Part model, mm, in its own coordinate system. Coordinates: 2 decimals unless noted, no trailing zeros. Order: outer loops, then holes, each group sorted by start corner. A loop starts at its lowest first (then second) coordinate and runs counter-clockwise, first axis right, second up.
1) Cut at A-A (x = 0). List the corners of the cut face in (y, z).
2) Cut at D-D (z = -25). List the corners of the cut face in (x, y).
3) Cut at C-C (z = 8.5). List the corners of the cut face in (x, y), and give its area (3 significant figures).
4) Cut at B-B (z = 0). List the corners of the cut face in (x, y), and give its area (3 significant figures).
5) Pin check, flat tips, straight feed: pin 1 Ø4 at (x, z) = (21.65, 12.5) entering from +Y; pin 2 Ø1 at (x, y) = (23.5, 0.5) entering from -Z; pin 3 Ø6 at (x, z) = (0, -15.25) entering from -Y. Stop position of each tip, or through.
6) Wall check: L1, parallel to X at y = 2.6, z = -14; L2, parallel to X at y = 0.8, z = 10.5; L3, parallel to Z at x = -11.5, y = 2.5. Give the ranges that are in metal, low to high.
```python
from build123d import *

# Parameters (mm, degrees)
SKETCH1_R           = 30
SKETCH1_R_2         = 17
BOSS_EXTRUDE1_DEPTH = 3
SKETCH2_R           = 4.75
SKETCH2_R_2         = 2.55
BOSS_EXTRUDE2_DEPTH = 3
SKETCH3_R           = 2.55
CUT_EXTRUDE1_DEPTH  = 43.532340636
CIRPATTERN1_COUNT   = 3
FILLET1_R           = 0.5
SKETCH4_R           = 2.55
CUT_EXTRUDE2_DEPTH  = 43.532340784
CIRPATTERN2_COUNT   = 3


with BuildPart() as part:
    # Sketch1 → Boss-Extrude1 (new body)
    with BuildSketch(Plane(origin=(0, 0, 0), x_dir=(1, 0, 0), z_dir=(0, 1, 0))):
        with Locations(Location((0, 0, 0), (0, 0, 270))):
            Circle(SKETCH1_R)
        with Locations(Location((0, 0, 0), (0, 0, 270))):
            Circle(SKETCH1_R_2, mode=Mode.SUBTRACT)
    extrude(amount=BOSS_EXTRUDE1_DEPTH)

    # Sketch2 → Boss-Extrude2 (add)
    with BuildSketch(Plane(origin=(0, 3, 0), x_dir=(1, 0, 0), z_dir=(0, 1, 0))):
        with Locations((0, 15.25)):
            Circle(SKETCH2_R)
        with Locations((0, 15.25)):
            Circle(SKETCH2_R_2, mode=Mode.SUBTRACT)
    boss_extrude2 = extrude(amount=-BOSS_EXTRUDE2_DEPTH)

    # Sketch3 → Cut-Extrude1 (cut, through all)
    with BuildSketch(Plane(origin=(0, 3, 0), x_dir=(1, 0, 0), z_dir=(0, 1, 0))):
        with Locations(Location((0, 15.25, 0), (0, 0, 270))):
            Circle(SKETCH3_R)
    cut_extrude1 = extrude(amount=-CUT_EXTRUDE1_DEPTH, mode=Mode.SUBTRACT)

    # CirPattern1: Boss-Extrude2, Cut-Extrude1 ×3 about axis
    cirpattern1_axis = Axis((0, 0, 0), (0, 1, 0))
    add([boss_extrude2.rotate(cirpattern1_axis, i * 360 / CIRPATTERN1_COUNT) for i in range(1, CIRPATTERN1_COUNT)])
    add([cut_extrude1.rotate(cirpattern1_axis, i * 360 / CIRPATTERN1_COUNT) for i in range(1, CIRPATTERN1_COUNT)], mode=Mode.SUBTRACT)

    # Fillet1
    fillet1_edges = [part.edges().sort_by_distance(p)[0] for p in [
        (-4.618326952, 1.5, -16.360655738),
        (4.618326952, 1.5, -16.360655738),
        (16.477906967, 1.5, 4.180739406),
        (11.859580016, 1.5, 12.179916332),
        (-16.477906967, 1.5, 4.180739406),
        (-11.859580016, 1.5, 12.179916332),
    ]]
    fillet(fillet1_edges, radius=FILLET1_R)

    # Sketch4 → Cut-Extrude2 (cut, through all)
    with BuildSketch(Plane(origin=(0, 3, 0), x_dir=(1, 0, 0), z_dir=(0, 1, 0))):
        with Locations(Location((0, 25, 0), (0, 0, 270))):
            Circle(SKETCH4_R)
    cut_extrude2 = extrude(amount=-CUT_EXTRUDE2_DEPTH, mode=Mode.SUBTRACT)

    # CirPattern2: Cut-Extrude2 ×3 about axis
    cirpattern2_axis = Axis((0, 0, 0), (0, 1, 0))
    for i in range(1, CIRPATTERN2_COUNT):
        add(cut_extrude2.rotate(cirpattern2_axis, i * 360 / CIRPATTERN2_COUNT), mode=Mode.SUBTRACT)


solid = part.part
```
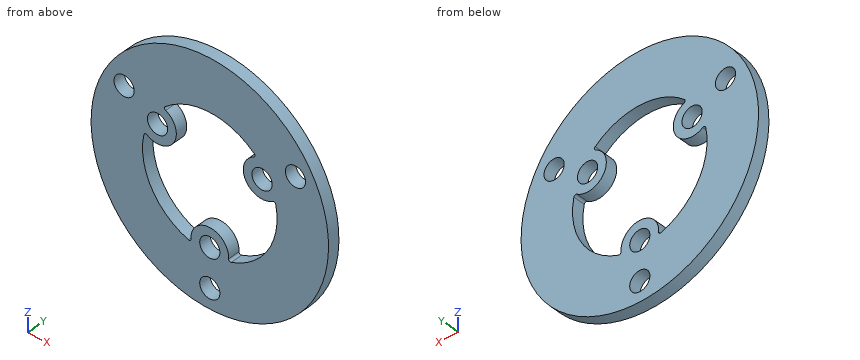
Geometry check:
1. outline: (0, -30) - (3, -30) - (3, -27.55) - (0, -27.55) - close; (0, -22.45) - (3, -22.45) - (3, -17.8) - (0, -17.8) - close; (0, -12.7) - (3, -12.7) - (3, -10.5) - (0, -10.5) - close; (0, 17) - (3, 17) - (3, 30) - (0, 30) - close
2. outline: (-16.58, 0) - (-2.55, 0) - (-2.55, 3) - (-16.58, 3) - close; (2.55, 0) - (16.58, 0) - (16.58, 3) - (2.55, 3) - close
3. outline: (-28.77, 0) - (-15.6, 0) - (-15.6, 3) - (-28.77, 3) - close; (-10.81, 0) - (-8.54, 0) - (-8.54, 3) - (-10.81, 3) - close; (8.54, 0) - (10.81, 0) - (10.81, 3) - (8.54, 3) - close; (15.6, 0) - (28.77, 0) - (28.77, 3) - (15.6, 3) - close
3. area: 92.7 mm2
4. outline: (-30, 0) - (-17, 0) - (-17, 3) - (-30, 3) - close; (17, 0) - (30, 0) - (30, 3) - (17, 3) - close
4. area: 78.0 mm2
5. pin 1: passes through
5. pin 2: stops at z = -19.26
5. pin 3: stops at y = 0
6. L1: x = -26.53 to -9.64, -4.58 to -2.22, 2.22 to 4.58, 9.64 to 26.53
6. L2: x = -28.1 to -23.23, -20.07 to -9.43, 9.43 to 20.07, 23.23 to 28.1
6. L3: z = -27.71 to -12.52, 3.19 to 5.73, 9.52 to 27.71
